Design review of the part built by this model. Coordinates are the model's own, in mm. Coordinates: 2 decimals unless noted, no trailing zeros. Order: outer loops, then holes, each group sorted by start corner. A loop starts at its lowest first (then second) coordinate and runs counter-clockwise, first axis right, second up. Notation, with made-up numbers: (51.5, 41) -> (67.5, 41) arc R5 ccw to (67.5, 49) -> close; hole circle Ø5 at (79, 47.5). An arc over 180 degrees is marked (long way). Write item = value, one per line.
Autodesk Inventor part; units mm, degrees
ref_plane "YZ Plane" through (0, 0, 0) normal (1, 0, 0) x (0, 1, 0)
ref_plane "XZ Plane" through (0, 0, 0) normal (0, 1, 0) x (-1, 0, 0)
ref_plane "XY Plane" through (0, 0, 0) normal (0, 0, 1) x (1, 0, 0)
sketch "Sketch1" plane through (0, 0, 0) normal (0, 1, 0) x (-1, 0, 0)
  circle A0 centre (0, 0) radius 2.1
  circle A1 centre (0, -25.4) radius 2.1
  circle A2 centre (-16.7115, 0) radius 1.5
  circle A3 centre (-16.7115, -10) radius 1.5
  circle A4 centre (0, 0) radius 5.275 construction
  circle A5 centre (0, -25.4) radius 5.275 construction
  circle A6 centre (-16.7115, 0) radius 4.675 construction
  circle A7 centre (-16.7115, -10) radius 4.675 construction
  line L0 (-0.1894, 5.2716) -> (-16.8793, 4.672)
  line L1 (5.275, 0) -> (5.275, -25.4)
  line L2 (-3.6758, -29.1834) -> (-19.9692, -13.353)
  line L3 (-21.3865, 0) -> (-21.3865, -10)
  arc A8 (-3.6758, -29.1834) -> (5.275, -25.4) centre (0, -25.4) ccw
  arc A9 (5.275, 0) -> (-0.1894, 5.2716) centre (0, 0) ccw
  arc A10 (-16.8793, 4.672) -> (-21.3865, 0) centre (-16.7115, 0) ccw
  arc A11 (-21.3865, -10) -> (-19.9692, -13.353) centre (-16.7115, -10) ccw
  dimension "d0" = 4.2
  dimension "d1" = 25.4
  dimension "d2" = 16.7115
  dimension "d3" = 3
  dimension "d4" = 10
  dimension "d5" = 3.175
  dimension "d6" = 3.175
extrude "Extrusion1" add sketch "Sketch1" along normal blind 4.5994
chamfer "Chamfer1" distance 0.1984 angle 45 2 edges at (18.2115, 0, 0) (18.2115, 0, -10)
chamfer "Chamfer2" distance 0.7937 angle 45 8 edges at (-2.0537, 4.5994, -30.2588) (-5.275, 4.5994, -12.7) (-3.6624, 4.5994, 3.7964) (8.5344, 4.5994, 4.9718) (20.076, 4.5994, 3.2458) (21.3865, 4.5994, -5) (21.0176, 4.5994, -11.8201) (11.8225, 4.5994, -21.2682)
equation "\"d6\" = d5"
properties part number "CNC-025-YAxisCableCarrierMount" material "ABS Plastic"
(1) We need section A-A (y = 0.85). Give the number of separate pieces and of enclosed holes in the cut face, and give its area (3 significant figures).
Report:
separate_pieces = 1
enclosed_holes = 4
area = 711 mm²
(2) The part is to be moulded in two halves that separate along Z. For faces 1 (the flat face through (5, 4.599, -9)), 2 (the cylindrical face through (-2.133, 1.876, -30.224)), 3 (the cylindrical face through (-1.13, 2.27, -27.17)), 4 (the conical face through (-3.17, 4.46, 3.36)), say which applies: released by +Z, released by -Z, zero draft, split by the parting line, or undercut.
Report:
face_1 = zero draft
face_2 = released by -Z
face_3 = undercut
face_4 = released by +Z
(3) We need section B-B (z = -24.5). Write out the cut boundary in (x, y) (3 decimals), and give its area (3 significant figures).
Report:
outline = (-5.275, 0) -> (-1.897, 0) -> (-1.897, 4.599) -> (-4.481, 4.599) -> (-5.275, 3.806) -> close; (1.897, 0) -> (8.496, 0) -> (8.496, 3.806) -> (7.357, 4.599) -> (1.897, 4.599) -> close
area = 45.1 mm²
(4) We need section C-C (x = 12.25). Write out the cut boundary in (y, z), and give its area (3 significant figures).
Report:
outline = (0, -20.85) -> (3.81, -20.85) -> (4.6, -19.75) -> (4.6, 4.04) -> (3.81, 4.84) -> (0, 4.84) -> close
area = 117 mm²
(5) Insertion check: pin 1 (1.5 mm diameter, centred on x = 12, y = 2, fed in from +Z); pin 2 (1 mm diameter, centred on x = 6.5, y = 2.5, fed in from +Z). Each pin has a flat end and moves straight along its axis. Give the tip position at first contact, or say it passes through.
Report:
pin_1 = 4.87
pin_2 = 5.06
(6) For L1, parallel to Z at x = 16, y = 1.6; L2, parallel to Z at x = 1, y = 2.2; L3, parallel to X at y = 1.3, z = 4, list the stretches that pass through material, from the lowest coordinate up.
Report:
L1 = -17.21 to -11.32, -8.68 to -1.32, 1.32 to 4.7
L2 = -30.58 to -27.25, -23.55 to -1.85, 1.85 to 5.24
L3 = -3.44 to 19.13
